Design review of the part shown in the three views and the two pictorial views. Dimensions are in mm from the part's minimum x, y and z. A direction names the side the tool comes from. Round coordinates to 2 decimals unless told otherwise and drop trailing zeros. Write each loop counter-clockwise with the first axis right and the second up, starting at its lowest first coordinate (ties: lowest second). Pieces come first, ordered by that corner, then holes. Notation, with made-up numbers: (-32, 58.25) - (27, 58.25) arc R20 ccw to (27, 71.25) - close; hole circle Ø5 at (-33, 38). An arc over 180 degrees is marked (long way). One line per item, written item: value. Start each with the question number.
Q1. Add section B-B on y = 683.5. Write out the cut boundary in (x, z).
Q2. Add section A-A on z = 106.5. Write out the cut boundary in (x, y), and give its area (3 significant figures).
Q3. Clearance check with flat-ended pins moving along their axes: pin 1 Ø10 at (y, z) = (876, 111) entering from +X; pin 2 Ø1 at (x, z) = (371, 432) entering from +Y; pin 3 Ø1 at (y, z) = (200.5, 486) entering from -X. State where each tip first meets the part, or that it passes through.
Q4. For probe 1 along X at (y, z) = (391, 213); probe 2 along X at (y, z) = (947, 375), list the stretches that pass through material, from the lowest coordinate up.
Q5. Mouldability with a two-part tool opening along X and no side actions: class the marked faces 4, 5 and 6 as +X half, -X half, draft (parallel to the pull), parting line (faces both ways), or undercut.
Q6. Add section D-D on z = 874. Write out the cut boundary in (x, y), and give its area (3 significant figures).
Q7. Tool access review of the marked faces 1, 2 and 3: name each direction out of +Z, -Z, +X, -X, +Y, -Y from which nothing blocks a thin tool from reaching the whole face with its end or side.
Q8. Add section C-C on x = 746. Write out the cut boundary in (y, z).
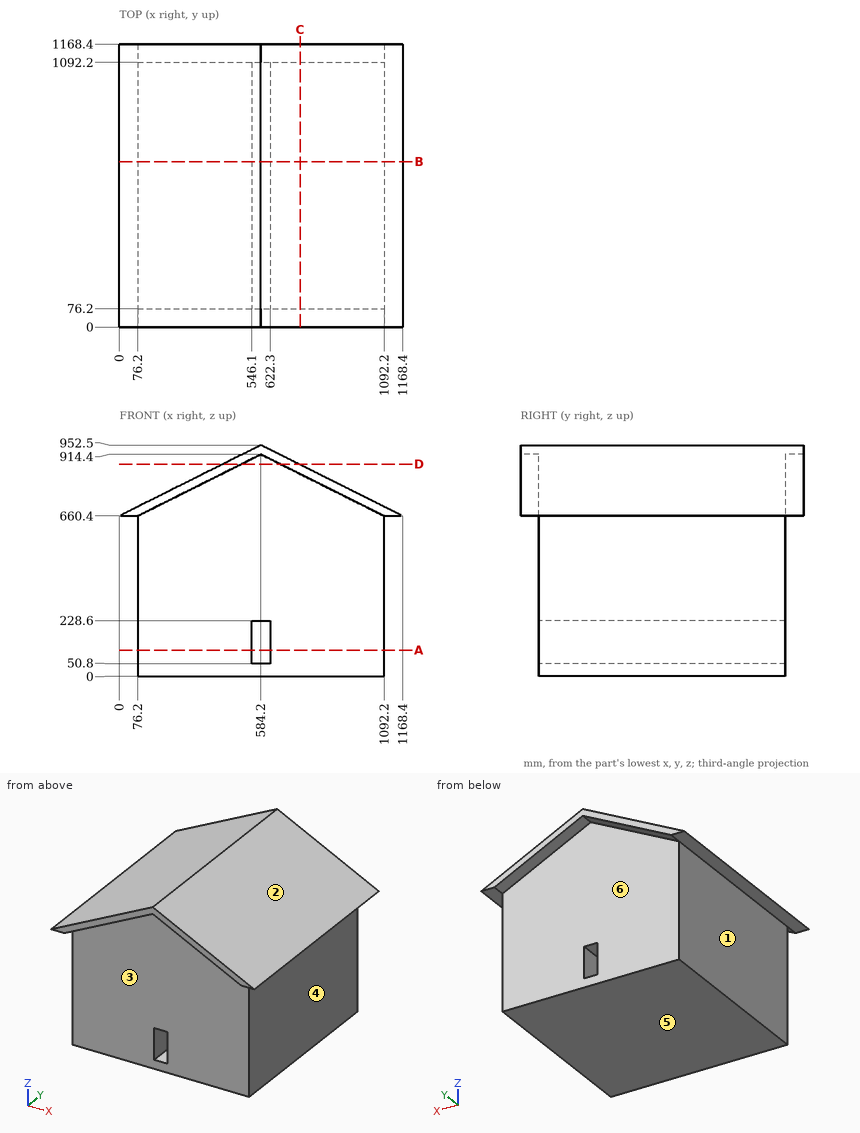
Result set:
1. outline: (0, 660.4) - (76.2, 660.4) - (76.2, 0) - (1092.2, 0) - (1092.2, 660.4) - (1168.4, 660.4) - (584.2, 952.5) - close; hole (546.1, 50.8) - (622.3, 50.8) - (622.3, 228.6) - (546.1, 228.6) - close
2. outline: (76.2, 76.2) - (546.1, 76.2) - (546.1, 1092.2) - (76.2, 1092.2) - close; (622.3, 76.2) - (1092.2, 76.2) - (1092.2, 1092.2) - (622.3, 1092.2) - close
2. area: 955,000 mm^2
3. pin 1: stops at x = 1092.2
3. pin 2: stops at y = 1092.2
3. pin 3: stops at x = 76.2
4. probe 1: x = 76.2 to 546.1, 622.3 to 1092.2
4. probe 2: x = 76.2 to 1092.2
5. face 4: +X half
5. face 5: draft
5. face 6: undercut
6. outline: (427.2, 0) - (503.4, 0) - (503.4, 76.2) - (665, 76.2) - (665, 0) - (741.2, 0) - (741.2, 1168.4) - (665, 1168.4) - (665, 1092.2) - (503.4, 1092.2) - (503.4, 1168.4) - (427.2, 1168.4) - close
6. area: 342,000 mm^2
7. face 1: -Z, -X, +Y, -Y
7. face 2: +Z, +X, +Y, -Y
7. face 3: -Z, -Y
8. outline: (0, 833.5) - (76.2, 833.5) - (76.2, 0) - (1092.2, 0) - (1092.2, 833.5) - (1168.4, 833.5) - (1168.4, 871.6) - (0, 871.6) - close
